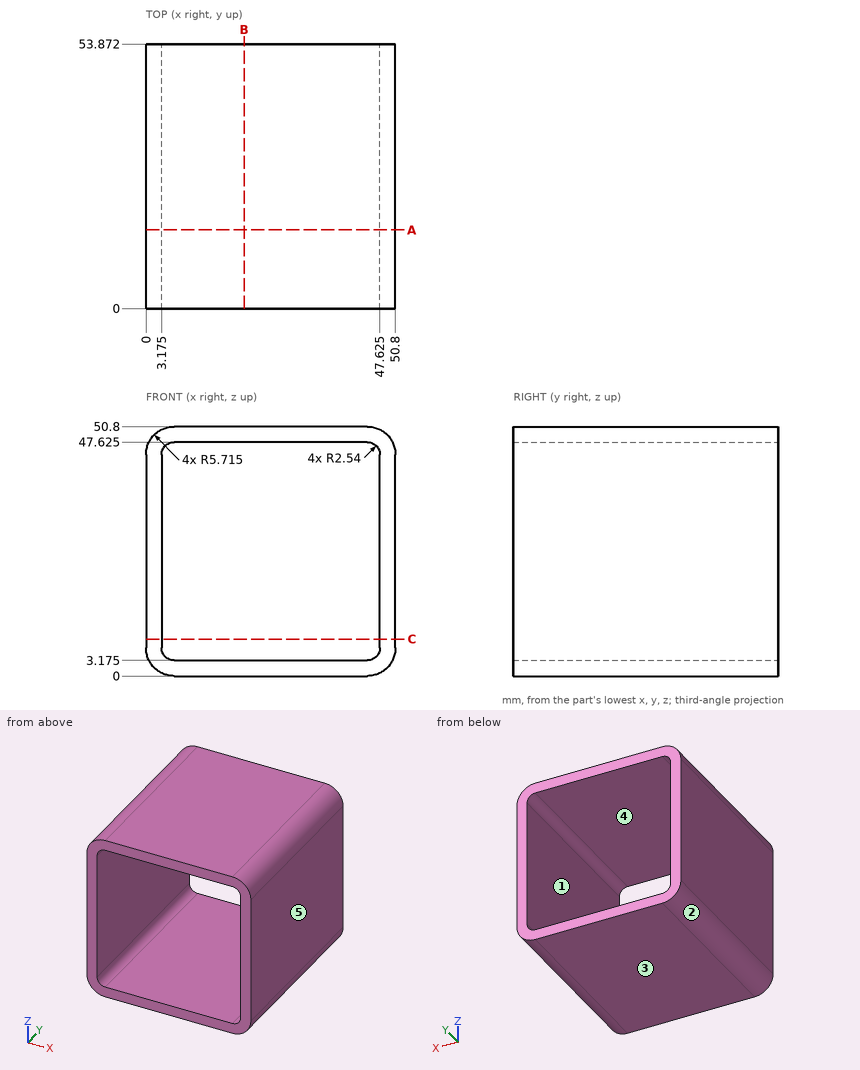
Part print with two shaded views. Sizes in mm from the minimum x, y, z corner. A direction names the side the tool comes from. Coordinates: 2 decimals unless noted, no trailing zeros. Write each loop counter-clockwise with the first axis right and the second up, starting at its lowest first coordinate (ties: lowest second). Pieces come first, ordered by that corner, then holes. Notation, with made-up numbers: (0.5, -18) - (32.5, -18) arc R30 ccw to (32.5, 5) - close; hole circle Ø10 at (-26, 79.25). An arc over 180 degrees is marked (long way). One line per item, written item: value. Start each with the question number.
1. Slice it at B-B (x = 20). Write the cut outline in (y, z) (1 decimal), plus the area to 3 significant figures.
2. Slice it at C-C (z = 7.5). Write the cut outline in (x, y) (1 decimal), plus the area to 3 significant figures.
3. Probe line 1 (Z direction, x = 12, y = 7.5) (1 decimal); line 2 (X direction, y = 14.5, z = 4.5) (1 decimal). List the from-to ranges inside material, lowest first. Write a range as from..to.
4. Tool access for the marked faces 1 and 2: list every direction of +Z, -Z, +X, -X, +Y, -Y with a clear straight run to the whole face (end or side of a thin tool).
5. Mould opens along X. For the marked faces 3, 4 and 5 say: released by +X, released by -X, zero draft, split by the parting line, or undercut.
6. Slice it at A-A (y = 16). Write the cut outline in (x, z) (1 decimal).
Answers below:
1. outline: (0, 0) - (53.9, 0) - (53.9, 3.2) - (0, 3.2) - close; (0, 47.6) - (53.9, 47.6) - (53.9, 50.8) - (0, 50.8) - close
1. area: 342 mm^2
2. outline: (0, 0) - (3.2, 0) - (3.2, 53.9) - (0, 53.9) - close; (47.6, 0) - (50.8, 0) - (50.8, 53.9) - (47.6, 53.9) - close
2. area: 342 mm^2
3. line 1: z = 0..3.2, 47.6..50.8
3. line 2: x = 0.1..3.5, 47.3..50.7
4. face 1: +Y, -Y
4. face 2: -Z, -X, +Y, -Y
5. face 3: zero draft
5. face 4: undercut
5. face 5: released by +X
6. outline: (0, 5.7) arc R5.7 ccw to (5.7, 0) - (45.1, 0) arc R5.7 ccw to (50.8, 5.7) - (50.8, 45.1) arc R5.7 ccw to (45.1, 50.8) - (5.7, 50.8) arc R5.7 ccw to (0, 45.1) - close; hole (3.2, 5.7) arc R2.5 ccw to (5.7, 3.2) - (45.1, 3.2) arc R2.5 ccw to (47.6, 5.7) - (47.6, 45.1) arc R2.5 ccw to (45.1, 47.6) - (5.7, 47.6) arc R2.5 ccw to (3.2, 45.1) - close
